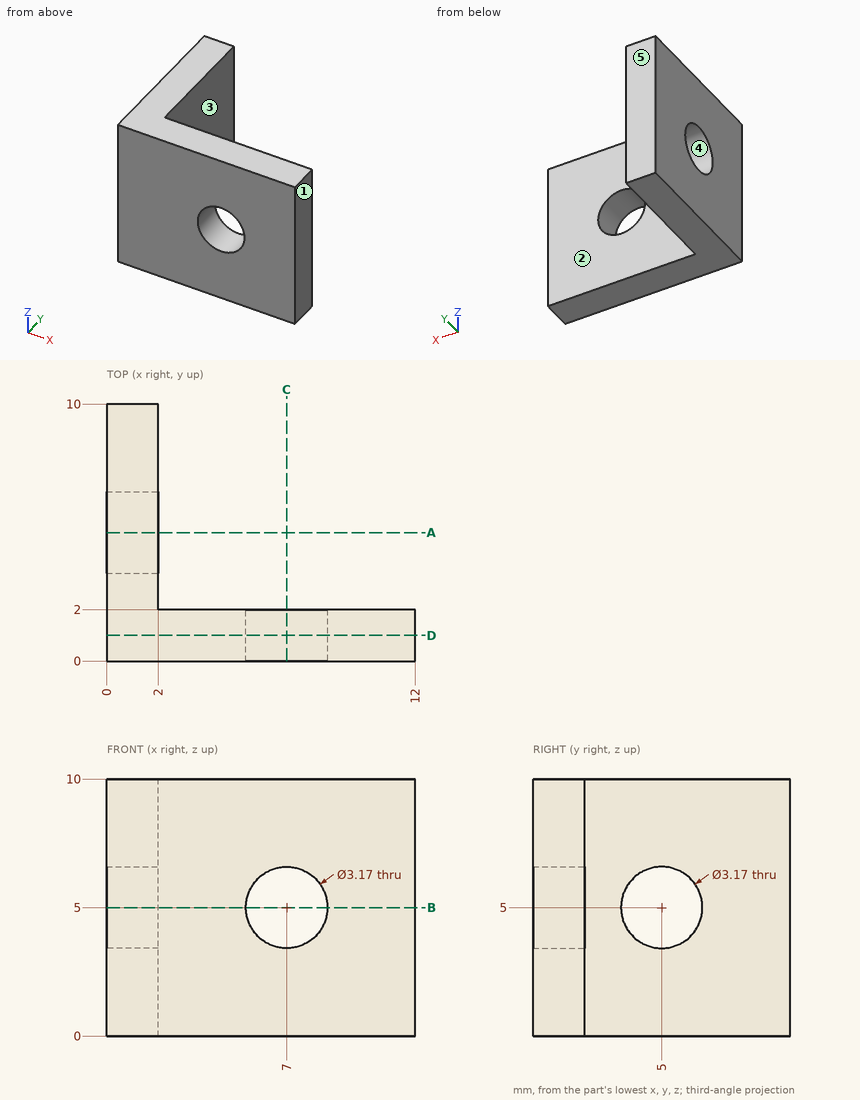
Geometry: see drawing. Coordinates: mm, zero at the bounding-box minimum. A direction names the side the tool comes from. Coordinates: 2 decimals unless noted, no trailing zeros. Write each loop counter-clockwise with the first axis right and the second up, starting at its lowest first coordinate (ties: lowest second). Pieces come first, ordered by that corner, then holes.
1) Mould query, pull axis Y, two halves, no side actions, for the marked faces 3, 4 and 5. Classes: pulls with the +Y half, pulls with the -Y half, needs draft (parallel to the pull), parting line crosses it, or undercut.
2) Pin query (flat end, axial travel): pin 1 Ø3 at (x, z) = (8, 6) entering from +Y; pin 2 Ø2.5 at (y, z) = (7, 7) entering from +X. Return the tip coordinate at first contact, or that it passes through.
3) Set-up query: the marked faces 1 and 2. Return all of +Z, -Z, +X, -X, +Y, -Y with unobstructed straight access to the full face (end or side cutting, diameter ignored); none if empty.
4) Section D-D on y = 1. Output: boundary loops of the cut face in (x, z) (3 decimals).
5) Material intervals for line 1 along Y through (x, z) = (0.9, 5) (3 decimals); line 2 along X through (y, z) = (6.5, 8.5), sorted ascending.
6) Section B-B on z = 5. Output: boundary loops of the cut face in (x, y) (3 decimals), and give its area (3 significant figures).
7) Section A-A on y = 5. Output: boundary loops of the cut face in (x, z) (3 decimals).
Check result:
1. face 3: needs draft
1. face 4: undercut
1. face 5: pulls with the +Y half
2. pin 1: stops at y = 2
2. pin 2: stops at x = 2
3. face 1: +Z, -Z, +X, +Y, -Y
3. face 2: +Z, -Z, +X, +Y
4. outline: (0, 0) - (12, 0) - (12, 10) - (0, 10) - close; hole circle Ø3.17 at (7, 5)
5. line 1: y = 0 to 3.415, 6.585 to 10
5. line 2: x = 0 to 2
6. outline: (0, 0) - (5.415, 0) - (5.415, 2) - (2, 2) - (2, 3.415) - (0, 3.415) - close; (0, 6.585) - (2, 6.585) - (2, 10) - (0, 10) - close; (8.585, 0) - (12, 0) - (12, 2) - (8.585, 2) - close
6. area: 27.3 mm2
7. outline: (0, 0) - (2, 0) - (2, 3.415) - (0, 3.415) - close; (0, 6.585) - (2, 6.585) - (2, 10) - (0, 10) - close
